```python
from build123d import *

# Parameters (mm, degrees)
F0_W     = 12.7
F0_H     = 76.2
F1_DEPTH = 50.8
F3_DEPTH = 12.7


# Not quite as in the source:
# - a pattern or mirror of a feature is missing from the dataset's text; its kind, count and spacing are read off the source's solid


with BuildPart() as f1:
    # F0 (on Right) → F1 (new body, symmetric)
    with BuildSketch(Plane.YZ):
        Rectangle(F0_W, F0_H)
    extrude(amount=F1_DEPTH, both=True)

    # F2 (on face) → F3 (cut)
    with BuildSketch(Plane(origin=(-50.8, 0, 0), x_dir=(0, -1, 0), z_dir=(-1, 0, 0))):
        Polygon((6.35, -26.0372895852), (6.35, 26.0372895852), (-6.35, 28.575), (-6.35, -28.575), align=None)
    f3 = extrude(amount=-F3_DEPTH, mode=Mode.SUBTRACT)

    # F3_copies: F3 across plane
    add(f3.mirror(Plane(origin=(0, 0, 0), x_dir=(0, 0, 1), z_dir=(1, 0, 0))), mode=Mode.SUBTRACT)


solid = f1.part
```
Here's how the part is built. I have some questions about the finished solid (model axes, mm). A direction names the side the tool comes from. Round coordinates to 2 decimals unless told otherwise and drop trailing zeros. Order: outer loops, then holes, each group sorted by start corner. A loop starts at its lowest first (then second) coordinate and runs counter-clockwise, first axis right, second up. Notation, with made-up numbers: (84.5, 28) -> (133.5, 28) arc R18 ccw to (133.5, 63) -> close; hole circle Ø2 at (36.25, -7). An arc over 180 degrees is marked (long way). Use a Markdown table: item, result. Add a question column.
(1) Suppose I cut it at C-C, the plane z = 9.5. Please give me the cut outline in (x, y).
(2) I need wall thicknesses on line 1 along X through (y, z) = (1.5, 21); line 2 along Z through (x, y) = (43.5, -1); line 3 along Z through (x, y) = (-42.5, 5.25). Which ranges of each line are inside material? Lowest first, please.
(3) If we mould it in two halves opening along Z, with no side actions, what happens to faces 1 (the face through (1, 0, 38.1)), 2 (the face through (50.8, 0, -32)), 3 (the face through (38.1, 0, 0))? For each: released by +Z, released by -Z, zero draft, split by the parting line, or undercut.
(4) For faces 4 (the face through (44.539, 0.089, -27.324)), 5 (the face through (1, -6.35, -1)), 6 (the face through (-44.54, -0.09, 27.29)), which set-ups out of +Z, -Z, +X, -X, +Y, -Y let a thin tool reach every point of the face, with its end or its side?
(5) Suppose I cut it at B-B, the plane y = -3.5. Please give me the cut outline in (x, z), and give its area (3 significant figures).
(6) Suppose I cut it at A-A, the plane x = 45.5. Please give me the cut outline in (y, z) (3 decimals).
(7) Suppose I cut it at D-D, the plane y = 1. Please give me the cut outline in (x, z), and give its area (3 significant figures).
(8) For pin 1 Ø4 at (y, z) = (3, -1) entering from -X; pin 2 Ø6 at (y, z) = (-0.5, 8) entering from +X, each with a flat end and sliding along its axis, tell me the tip position at first contact or that it passes through.
Verdict:
| question | item | result |
|---|---|---|
| 1 | outline | (-38.1, -6.35) -> (38.1, -6.35) -> (38.1, 6.35) -> (-38.1, 6.35) -> close |
| 2 | line 1 | -38.1 to 38.1 |
| 2 | line 2 | -38.1 to -27.11, 27.11 to 38.1 |
| 2 | line 3 | -38.1 to -28.36, 28.36 to 38.1 |
| 3 | face 1 | released by +Z |
| 3 | face 2 | zero draft |
| 3 | face 3 | undercut |
| 4 | face 4 | +X, +Y |
| 4 | face 5 | +Z, -Z, +X, -X, -Y |
| 4 | face 6 | -X, +Y |
| 5 | outline | (-50.8, -38.1) -> (50.8, -38.1) -> (50.8, -26.61) -> (38.1, -26.61) -> (38.1, 26.61) -> (50.8, 26.61) -> (50.8, 38.1) -> (-50.8, 38.1) -> (-50.8, 26.61) -> (-38.1, 26.61) -> (-38.1, -26.61) -> (-50.8, -26.61) -> close |
| 5 | area | 6,390 mm2 |
| 6 | outline | (-6.35, -38.1) -> (6.35, -38.1) -> (6.35, -28.575) -> (-6.35, -26.037) -> close; (-6.35, 26.037) -> (6.35, 28.575) -> (6.35, 38.1) -> (-6.35, 38.1) -> close |
| 7 | outline | (-50.8, -38.1) -> (50.8, -38.1) -> (50.8, -27.51) -> (38.1, -27.51) -> (38.1, 27.51) -> (50.8, 27.51) -> (50.8, 38.1) -> (-50.8, 38.1) -> (-50.8, 27.51) -> (-38.1, 27.51) -> (-38.1, -27.51) -> (-50.8, -27.51) -> close |
| 7 | area | 6,340 mm2 |
| 8 | pin 1 | x = -38.1 |
| 8 | pin 2 | x = 38.1 |
